Part model, mm, in its own coordinate system. A direction names the side the tool comes from. Coordinates: 2 decimals unless noted, no trailing zeros. Loops run counter-clockwise (first coordinate to the right, second up) from the corner with the lowest first, then second, coordinate; pieces in that order, holes last. Notation, with made-up numbers: M 77,73.5 L 89,73.5 A16 ccw 89,94.5 Z; hole C -4.75,-22.75 d6. An arc over 180 degrees is marked long. Answer as a JSON object with one key per item and string values. Group by question number.
1. Mould opens along Y. For faces 3 (the face through (49.325, 10.055, 0.986)), 4 (the face through (9.95, -5.07, 0.99)), 5 (the face through (36.978, -5.466, 0.986)), 6 (the face through (58.17, -1.95, 0.99)) say: released by +Y, released by -Y, zero draft, split by the parting line, or undercut.
2. Drop flat-ended pins along their axis: pin 1 Ø6.5 at (x, y) = (50, 0) entering from -Z; pin 2 Ø0.6 at (x, z) = (-28.5, 1) entering from +Y; pin 3 Ø1 at (y, z) = (-2, 0.5) entering from +X. Give the stop position or say it passes through.
3. 3-axis set-ups, long thin cutter, end or side, ignore diameter. For faces 1 (the face through (-26, 8.5, 1)), 2 (the face through (27, 13, 1)): which of +Z, -Z, +X, -X, +Y, -Y reach the whole face in a straight line?
4. Saw through at C-C on x = -25.5. Write the cut outline in (y, z), then the cut area to 3 significant figures.
5. Drill centre lines: L1, parallel to Y at x = -50, z = 1.5; L2, parallel to X at y = -5.25, z = 1.3; L3, parallel to X at y = -3, z = 0.9. Where is each one in solid material? Low to high.
6. Saw through at B-B on z = 1.3. Write the cut outline in (x, y), then the cut area to 3 significant figures.
7. Saw through at A-A on y = 0. Write the cut outline in (x, z), then the cut area to 3 significant figures.
8. Saw through at D-D on y = 5.25. Write the cut outline in (x, z).
Autodesk Inventor part; units mm, degrees
ref_plane "YZ Plane" through (0, 0, 0) normal (1, 0, 0) x (0, 1, 0)
ref_plane "XZ Plane" through (0, 0, 0) normal (0, 1, 0) x (-1, 0, 0)
ref_plane "XY Plane" through (0, 0, 0) normal (0, 0, 1) x (1, 0, 0)
sketch "スケッチ1" plane through (0, 0, 0) normal (0, 0, 1) x (1, 0, 0)
  line L0 (-50, 0) -> (50, 0) construction
  circle A0 centre (-50, 0) radius 4.05
  circle A1 centre (50, 0) radius 4.05
  line L1 (-50, 8.5) -> (43, 8.5)
  line L2 (-50, -8.5) -> (43, -8.5)
  arc A2 (-50, 8.5) -> (-50, -8.5) centre (-50, 0) ccw
  line L3 (43, -8.5) -> (50.119, -8.3992)
  line L4 (43, 8.5) -> (50.119, 8.3992)
  arc A3 (50.119, -8.3992) -> (50.119, 8.3992) centre (50, 0) ccw
  line L5 (9, -7.5) -> (38, -7.5) construction
  line L6 (38, -7.5) -> (38, -2.5) construction
  line L7 (38, -2.5) -> (9, -2.5) construction
  line L8 (9, -2.5) -> (9, -7.5) construction
  line L9 (9, -5) -> (38, -5) construction
  circle A4 centre (11.5, -5) radius 1.55
  line L10 (23.5, -5) -> (23.5, -2.5) construction
  line L11 (44.1615, 13) -> (9.1615, 13)
  line L12 (9.1615, 13) -> (-0.8385, 8.5)
  line L13 (44.1615, 13) -> (54.1615, 7.2967)
  circle A5 centre (35.5, -5) radius 1.55
  point P0 (0, 0)
  point P1 (0, 0)
  point P2 (52.0517, 8.5)
  dimension "d0" = 100
  dimension "d1" = 8.1
  dimension "d2" = 8.5
  dimension "d8" = 8.1
  dimension "d9" = 7
  dimension "d10" = 8.4
  dimension "d12" = 5
  dimension "d13" = 29
  dimension "d15" = 2.5
  dimension "d17" = 13
  dimension "d19" = 10
  dimension "d20" = 35
  dimension "d25" = 12
  dimension "d26" = 10
  dimension "d34" = 1
  dimension "d35" = 3.1
extrude "押し出し1" add sketch "スケッチ1" along normal blind 2
fillet "フィレット1" radius 2 3 edges at (-0.8385, 8.5, 1) (9.1615, 13, 1) (44.1615, 13, 1)
equation "\"d8\" = d1"
equation "\"d19\" = d18"
equation "\"d26\" = d19"
properties part number "リンク_メインフレーム_6_3" material "GFRP"
Outcome:
{
 "1": {"face 3": "released by +Y", "face 4": "undercut", "face 5": "undercut", "face 6": "split by the parting line"},
 "2": {"pin 1": "passes through", "pin 2": "stops at y = 8.5", "pin 3": "stops at x = 58.27"},
 "3": {"face 1": "+Z, -Z, -X, +Y", "face 2": "+Z, -Z, +X, -X, +Y"},
 "4": {"outline": "M -8.5,0 L 8.5,0 L 8.5,2 L -8.5,2 Z", "area": "34.0 mm²"},
 "5": {"L1": "y = -8.5 to -4.05, 4.05 to 8.5", "L2": "x = -56.68 to 9.97, 13.03 to 33.97, 37.03 to 56.56", "L3": "x = -57.95 to -52.72, -47.28 to 47.28, 52.72 to 57.85"},
 "6": {"outline": "M -50,-8.5 L 43,-8.5 L 50.12,-8.4 A8.4 ccw 54.16,7.3 L 44.62,12.74 A2 ccw 43.63,13 L 9.59,13 A2 ccw 8.77,12.82 L -0.45,8.68 A2 cw -1.27,8.5 L -50,8.5 A8.5 ccw Z; hole C -50,0 d8.1; hole C 11.5,-5 d3.1; hole C 35.5,-5 d3.1; hole C 50,0 d8.1", "area": "2,000 mm²"},
 "7": {"outline": "M -58.5,0 L -54.05,0 L -54.05,2 L -58.5,2 Z; M -45.95,0 L 45.95,0 L 45.95,2 L -45.95,2 Z; M 54.05,0 L 58.4,0 L 58.4,2 L 54.05,2 Z", "area": "201 mm²"},
 "8": {"outline": "M -56.68,0 L 56.56,0 L 56.56,2 L -56.68,2 Z"}
}
